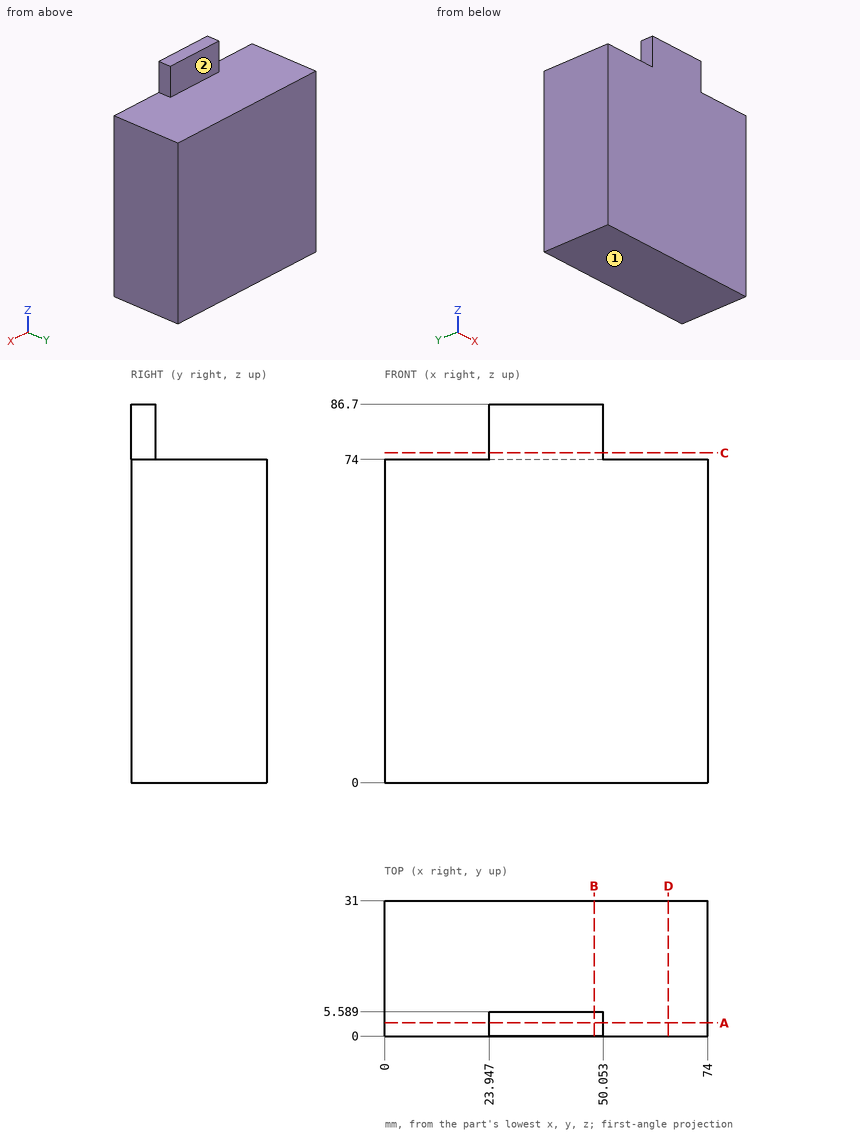
Study the drawing (mm; zero at the part's minimum x, y, z) and answer. A direction names the side the tool comes from. Give positions to 0.01 mm unless a question says otherwise; leave off trailing zeros. Write each loop counter-clockwise with the first axis right and the second up, starting at its lowest first coordinate (ties: lowest second). Pieces come first, ordered by that corner, then holes. Notation, with made-up numbers: (34.25, 4) - (62.25, 4) arc R31 ccw to (62.25, 40) - close; hole circle Ø6 at (19, 63.25). An arc over 180 degrees is marked (long way). Use CSV: the item, a comma, the result in double quotes. Start each with the question number.
(1) Find section A-A (y = 3). Give the vertices of the cut face in (x, z).
(2) Find section B-B (x = 48). Give the vertices of the cut face in (y, z), plus the area to 4 significant figures.
(3) For the marked faces 1 and 2, determine the directions among +Z, -Z, +X, -X, +Y, -Y from which every point of the face is accessible in a straight line to the end or side of a thin tool.
(4) Find section D-D (x = 65). Give the vertices of the cut face in (y, z), plus the area to 3 significant figures.
(5) Given P1, Ø1.7, axis at y = 1.5, z = 78.5, coming from the -X side; P2, Ø9.5, axis at x = 30.5, y = 13.5, coming from the +Z side; P3, Ø4, axis at x = 36.5, z = 81, coming from the +Y side, each flat-ended and moving along its own axis, determine where each tip first touches the part or whether it passes through.
(6) Consider line 1 along Z through (x, y) = (40.5, 26); line 2 along X through (y, z) = (1, 81); line 3 along Y through (x, z) = (30, 82.5). Determine where each line is inside the solid, lowest interval first.
(7) Find section C-C (z = 75.5). Give the vertices of the cut face in (x, y), plus the area to 3 significant figures.
Findings below:
1,outline,"(0, 0) - (74, 0) - (74, 74) - (50.05, 74) - (50.05, 86.7) - (23.95, 86.7) - (23.95, 74) - (0, 74) - close"
2,outline,"(0, 0) - (31, 0) - (31, 74) - (5.59, 74) - (5.59, 86.7) - (0, 86.7) - close"
2,area,"2,365 mm2"
3,face 1,"-Z, +X, -X, +Y, -Y"
3,face 2,"+Z, +X, -X, +Y"
4,outline,"(0, 0) - (31, 0) - (31, 74) - (0, 74) - close"
4,area,"2,290 mm2"
5,P1,"x = 23.95"
5,P2,"z = 74"
5,P3,"y = 5.59"
6,line 1,"0 to 74"
6,line 2,"23.95 to 50.05"
6,line 3,"0 to 5.59"
7,outline,"(23.95, 0) - (50.05, 0) - (50.05, 5.59) - (23.95, 5.59) - close"
7,area,"146 mm2"
